Input: part model. Units: mm. Frame: model coordinates. A direction names the side the tool comes from. Give positions to 0.01 mm unless a question says otherwise; leave off trailing zeros. Loops run counter-clockwise (first coordinate to the right, second up) from the corner with the lowest first, then second, coordinate; pieces in that order, holes last. Notation, with made-up numbers: M -2.5,58.25 L 21.5,58.25 A24 cw 21.5,85.25 Z; hole C 54,51.5 d9. An arc over 180 degrees is marked long. Answer as a JSON object with one key per item and string values. Group by question number.
```python
from build123d import *

# Parameters (mm, degrees)
EXTRUDE_1_DEPTH     = 60
SKETCH_2_R          = 2.6
CUT_EXTRUDE_1_DEPTH = 8
SKETCH_3_R          = 7.5
CUT_EXTRUDE_2_DEPTH = 6
FILLET_2_R          = 1.2
SKETCH_4_W          = 72.60588745
SKETCH_4_H          = 8
EXTRUDE_2_DEPTH     = 5
FILLET_3_R          = 1.2
CHAMFER_3_SIZE      = 2


with BuildPart() as part:
    # Эскиз1 → Бобышка-Вытянуть1 (new body)
    with BuildSketch(Plane.XY):
        Polygon((-30, 0), (30, 0), (38, 8), (-38, 8), align=None)
    extrude(amount=EXTRUDE_1_DEPTH)

    # Эскиз2 → Вырез-Вытянуть1 (cut)
    with BuildSketch(Plane(origin=(0, 8, 0), x_dir=(1, 0, 0), z_dir=(0, 1, 0))):
        with Locations(Location((0, -10, 0), (0, 0, 180))):
            Circle(SKETCH_2_R)
        with Locations(Location((0, -50, 0), (0, 0, 180))):
            Circle(SKETCH_2_R)
    extrude(amount=-CUT_EXTRUDE_1_DEPTH, mode=Mode.SUBTRACT)

    # Эскиз3 → Вырез-Вытянуть2 (cut)
    with BuildSketch(Plane(origin=(0, 8, 0), x_dir=(1, 0, 0), z_dir=(0, 1, 0))):
        with Locations(Location((0, -10, 0), (0, 0, 180))):
            Circle(SKETCH_3_R)
        with Locations(Location((0, -50, 0), (0, 0, 180))):
            Circle(SKETCH_3_R)
    extrude(amount=-CUT_EXTRUDE_2_DEPTH, mode=Mode.SUBTRACT)

    # Скругление2
    fillet_2_edges = [part.edges().sort_by_distance(p)[0] for p in [
        (-38, 8, 30),
        (38, 8, 30),
    ]]
    fillet(fillet_2_edges, radius=FILLET_2_R)

    # Эскиз4 → Бобышка-Вытянуть2 (add)
    with BuildSketch(Plane.XY.offset(60)):
        with Locations((0, 4)):
            Rectangle(SKETCH_4_W, SKETCH_4_H)
    extrude(amount=EXTRUDE_2_DEPTH)

    # Скругление3
    fillet_3_edges = [part.edges().sort_by_distance(p)[0] for p in [
        (36.302943725, 8, 62.5),
        (-36.302943725, 8, 62.5),
    ]]
    fillet(fillet_3_edges, radius=FILLET_3_R)

    # Фаска3
    chamfer_3_edges = [part.edges().sort_by_distance(p)[0] for p in [
        (7.5, 8, 10),
        (7.5, 8, 50),
    ]]
    chamfer(chamfer_3_edges, length=CHAMFER_3_SIZE)


solid = part.part
```
1. Material intervals for L1, parallel to Z at x = 0, y = 1.05; L2, parallel to Z at x = 0, y = 3.25; L3, parallel to Y at x = -3.5, z = 50, sorted ascending.
2. First-contact query: P1, Ø4.5, axis at x = 0.5, z = 48.5, coming from the +Y side; P2, Ø4, axis at y = 2.5, z = 28, coming from the +X side; P3, Ø4, axis at y = 4.5, z = 28, coming from the -X side; P4, Ø4, axis at x = 0, z = 10, coming from the -Y side (3 decimals). Flat tips, straight axial feed; report the tip coordinate or a pass-through.
3. Section B-B (z = 10). Output: boundary loops of the cut face in (x, y), then the cut area to 3 significant figures.
4. Reachability of faces 4 (the flat face through (-33, 3, 30)), 5 (the flat face through (0, 8, 32)), 6 (the cylindrical face through (1.63, 4.03, 2.68)), 7 (the cylindrical face through (36.22, 7.24, 30.42)), 8 (the flat face through (33, 3, 30)) from +Z, -Z, +X, -X, +Y, -Y: full face, straight path, thin tool, end or side. Return the list, or none.
5. Section A-A (x = 0). Output: boundary loops of the cut face in (y, z).
6. Section C-C (z = 26.5). Output: boundary loops of the cut face in (x, y).
7. Mould query, pull axis Z, two halves, no side actions, for faces 1 (the flat face through (-1, 4, 65)), 2 (the cylindrical face through (-36.22, 7.24, 30.42)), 3 (the cylindrical face through (0.56, 1.01, 47.46)). Classes: pulls with the +Z half, pulls with the -Z half, needs draft (parallel to the pull), parting line crosses it, or undercut.
Geometry results:
{
 "1": {"L1": "0 to 7.4, 12.6 to 47.4, 52.6 to 65", "L2": "0 to 2.5, 17.5 to 42.5, 57.5 to 65", "L3": "0 to 2"},
 "2": {"P1": "y = 2", "P2": "x = 34.5", "P3": "x = -36.26", "P4": "through"},
 "3": {"outline": "M -35.95,5.95 L -30,0 L -2.6,0 L -2.6,2 L -7.5,2 L -7.5,6 L -9.5,8 L -35.1,8 A1.2 ccw Z; M 2.6,0 L 30,0 L 35.95,5.95 A1.2 ccw 35.1,8 L 9.5,8 L 7.5,6 L 7.5,2 L 2.6,2 Z", "area": "436 mm2"},
 "4": {"face 4": "-Z, -X, -Y", "face 5": "+Z, -Z, +X, -X, +Y", "face 6": "+Y", "face 7": "-Z, +X", "face 8": "-Z, +X, -Y"},
 "5": {"outline": "M 0,0 L 8,0 L 8,0.5 L 6,2.5 L 2,2.5 L 2,7.4 L 0,7.4 Z; M 0,12.6 L 2,12.6 L 2,17.5 L 6,17.5 L 8,19.5 L 8,40.5 L 6,42.5 L 2,42.5 L 2,47.4 L 0,47.4 Z; M 0,52.6 L 2,52.6 L 2,57.5 L 6,57.5 L 8,59.5 L 8,65 L 0,65 Z"},
 "6": {"outline": "M -35.95,5.95 L -30,0 L 30,0 L 35.95,5.95 A1.2 ccw 35.1,8 L -35.1,8 A1.2 ccw Z"},
 "7": {"face 1": "pulls with the +Z half", "face 2": "needs draft", "face 3": "undercut"}
}
